The listing builds one solid part. Answer for the finished solid, in the listing's coordinates (mm). Coordinates: 2 decimals unless noted, no trailing zeros. Order: outer loops, then holes, each group sorted by start corner. A loop starts at its lowest first (then second) coordinate and runs counter-clockwise, first axis right, second up. Notation, with made-up numbers: (64.25, 24) -> (82.25, 24) arc R26 ccw to (82.25, 54) -> close; hole circle Ø11 at (17.5, 26). An arc over 180 degrees is marked (long way). Answer in a Markdown table with one row per item. Add a question column.
```python
from build123d import *

# Parameters (mm, degrees)
SKETCH2_W               = 563.63
SKETCH2_H               = 369.5
BOSS_EXTRUDE1_DEPTH     = 12.7
SKETCH3_W               = 45.5
SKETCH3_H               = 10
CUT_EXTRUDE2_DEPTH      = 1
CUT_EXTRUDE2_DEPTH_BACK = 13.7


with BuildPart() as part:
    # Sketch2 → Boss-Extrude1 (new body)
    with BuildSketch(Plane(origin=(0, 0, 0), x_dir=(1, 0, 0), z_dir=(0, 1, 0))):
        Rectangle(SKETCH2_W, SKETCH2_H)
    extrude(amount=BOSS_EXTRUDE1_DEPTH)

    # Sketch3 → Cut-Extrude2 (cut, two sides)
    with BuildSketch(Plane(origin=(0, 12.7, 0), x_dir=(1, 0, 0), z_dir=(0, 1, 0))) as cut_extrude2_sk:
        with Locations((-190.485755703, 142.5)):
            Rectangle(SKETCH3_W, SKETCH3_H)
        with Locations((0.170132064, 142.5)):
            Rectangle(SKETCH3_W, SKETCH3_H)
        with Locations((190.170132064, 142.5)):
            Rectangle(SKETCH3_W, SKETCH3_H)
        with Locations((94.514244297, -142.5)):
            Rectangle(SKETCH3_W, SKETCH3_H)
        with Locations((-94.829867936, -142.5)):
            Rectangle(SKETCH3_W, SKETCH3_H)
    extrude(amount=CUT_EXTRUDE2_DEPTH, mode=Mode.SUBTRACT)
    extrude(cut_extrude2_sk.sketch, amount=-CUT_EXTRUDE2_DEPTH_BACK, mode=Mode.SUBTRACT)


solid = part.part
```
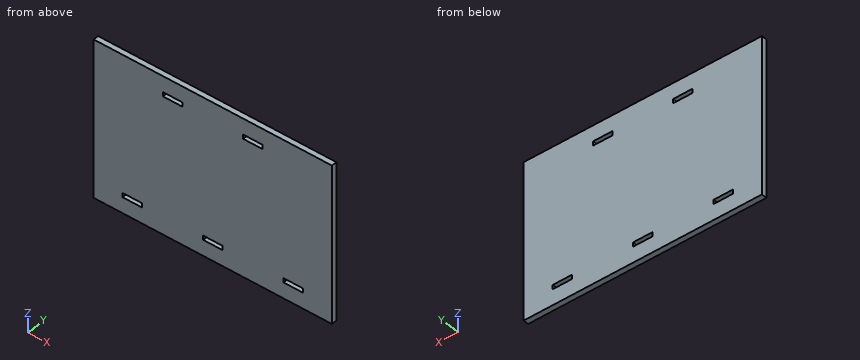
Q1. Straight lines are drawn through the part: line 1 (Z direction, x = -108.5, y = 5.75); line 2 (X direction, y = 12, z = -138.5) (3 decimals); line 3 (Z direction, x = -192.5, y = 2.75). For each, find the intervals that lie inside material, in ascending order.
Q2. A cutting plane is placed at A-A (x = 187.5). Determine the outline of the cut face in (y, z), then the cut area to 3 significant figures.
Q3. Given pin 1 (1 mm diameter, centred on x = 141, z = -82.5, fed in from -Y), flat-ended and moving along its own axis, determine where the tip first touches the part or whether it passes through.
Returned:
| question | item | result |
|---|---|---|
| 1 | line 1 | z = -184.75 to 137.5, 147.5 to 184.75 |
| 1 | line 2 | x = -281.815 to -213.236, -167.736 to -22.58, 22.92 to 167.42, 212.92 to 281.815 |
| 1 | line 3 | z = -184.75 to -147.5, -137.5 to 184.75 |
| 2 | outline | (0, -184.75) -> (12.7, -184.75) -> (12.7, -147.5) -> (0, -147.5) -> close; (0, -137.5) -> (12.7, -137.5) -> (12.7, 184.75) -> (0, 184.75) -> close |
| 2 | area | 4,570 mm² |
| 3 | pin 1 | stops at y = 0 |
